```python
from build123d import *

# Parameters (mm, degrees)
BOSS_EXTRUDE1_DEPTH = 40
SKETCH2_R           = 7.5
BOSS_EXTRUDE2_DEPTH = 5
FILLET1_R           = 10


with BuildPart() as part:
    # Sketch1 → Boss-Extrude1 (new, symmetric)
    with BuildSketch(Plane.XY):
        with BuildLine():
            Line((-42.261826174, 90.630778704), (0, 0))
            Line((0, 0), (57.1, 0))
            Line((57.1, 0), (78.545069205, 10))
            Line((78.545069205, 10), (70.06731645, 28.180599453))
            ThreePointArc((70.06731645, 28.180599453), (58.907926391, 38.47561206), (43.733601964, 37.96654498))
            Line((43.733601964, 37.96654498), (15.92675652, 25))
            Line((15.92675652, 25), (-11.151766263, 83.070079506))
            ThreePointArc((-11.151766263, 83.070079506), (-22.437519138, 93.411566687), (-37.730287239, 92.743870012))
            Line((-37.730287239, 92.743870012), (-42.261826174, 90.630778704))
        make_face()
    extrude(amount=BOSS_EXTRUDE1_DEPTH, both=True)

    # Sketch2 → Boss-Extrude2 (add, symmetric)
    with BuildSketch(Plane.XZ):
        with Locations(Location((30, 0, 0), (0, 0, 90))):
            Circle(SKETCH2_R)
    extrude(amount=BOSS_EXTRUDE2_DEPTH, both=True)

    # Fillet1
    # the kernel refuses this fillet: 10 mm, written as the material it takes off along each edge
    with BuildSketch(Plane(origin=(43.733601964, 37.96654498, -40), x_dir=(0.42261826174070133, -0.9063077870366492, 0), z_dir=(-0.9063077870366492, -0.4226182617407013, 0))) as fillet1_piece_1:
        with BuildLine():
            CenterArc((FILLET1_R, FILLET1_R), FILLET1_R, 180, 90)
            Line((0, FILLET1_R), (0, 0))
            Line((0, 0), (FILLET1_R, 0))
        make_face()
    extrude(amount=30.681459259, mode=Mode.SUBTRACT)
    with BuildSketch(Plane(origin=(51.94116071, 19.728234218, -40), x_dir=(0.9063077870366498, 0.42261826174069983, 0), z_dir=(0.42261826174069983, -0.9063077870366498, 0))) as fillet1_piece_2:
        with BuildLine():
            CenterArc((20 - FILLET1_R, FILLET1_R), FILLET1_R, 270, 90)
            Line((20, FILLET1_R), (20, 0))
            Line((20, 0), (20 - FILLET1_R, 0))
        make_face()
    revolve(axis=Axis((51.94116071, 19.728234218, -40), (0, 0, 1)), revolution_arc=89.228578439, mode=Mode.SUBTRACT)
    with BuildSketch(Plane(origin=(89.110525749, -12.657694676, -40), x_dir=(-0.90630778703665, -0.4226182617406995, 0), z_dir=(-0.42261826174069944, 0.9063077870366499, 0))) as fillet1_piece_3:
        with BuildLine():
            CenterArc((FILLET1_R, FILLET1_R), FILLET1_R, 180, 90)
            Line((0, FILLET1_R), (0, 0))
            Line((0, 0), (FILLET1_R, 0))
        make_face()
    extrude(amount=45.06007199, mode=Mode.SUBTRACT)
    with BuildSketch(Plane(origin=(-37.730287239, 92.743870012, -40), x_dir=(0.4226182617406985, -0.9063077870366504, 0), z_dir=(-0.9063077870366504, -0.42261826174069855, 0))) as fillet1_piece_4:
        with BuildLine():
            CenterArc((FILLET1_R, FILLET1_R), FILLET1_R, 180, 90)
            Line((0, FILLET1_R), (0, 0))
            Line((0, 0), (FILLET1_R, 0))
        make_face()
    extrude(amount=30, mode=Mode.SUBTRACT)
    with BuildSketch(Plane(origin=(89.110525749, -12.657694676, 40), x_dir=(-0.90630778703665, -0.4226182617406995, 0), z_dir=(-0.42261826174069944, 0.9063077870366499, 0))) as fillet1_piece_5:
        with BuildLine():
            CenterArc((FILLET1_R, -FILLET1_R), FILLET1_R, 90, 90)
            Line((0, -FILLET1_R), (0, 0))
            Line((0, 0), (FILLET1_R, 0))
        make_face()
    extrude(amount=45.06007199, mode=Mode.SUBTRACT)
    with BuildSketch(Plane(origin=(51.94116071, 19.728234218, 40), x_dir=(0.9063077870366498, 0.42261826174069983, 0), z_dir=(0.42261826174069983, -0.9063077870366498, 0))) as fillet1_piece_6:
        with BuildLine():
            CenterArc((20 - FILLET1_R, -FILLET1_R), FILLET1_R, 0, 90)
            Line((20, -FILLET1_R), (20, 0))
            Line((20, 0), (20 - FILLET1_R, 0))
        make_face()
    revolve(axis=Axis((51.94116071, 19.728234218, 40), (0, 0, 1)), revolution_arc=89.228578439, mode=Mode.SUBTRACT)
    with BuildSketch(Plane(origin=(43.733601964, 37.96654498, 40), x_dir=(0.42261826174070133, -0.9063077870366492, 0), z_dir=(-0.9063077870366492, -0.4226182617407013, 0))) as fillet1_piece_7:
        with BuildLine():
            CenterArc((FILLET1_R, -FILLET1_R), FILLET1_R, 90, 90)
            Line((0, -FILLET1_R), (0, 0))
            Line((0, 0), (FILLET1_R, 0))
        make_face()
    extrude(amount=30.681459259, mode=Mode.SUBTRACT)
    with BuildSketch(Plane(origin=(15.92675652, 25, 40), x_dir=(-0.9063077870366495, -0.42261826174070066, 0), z_dir=(-0.42261826174070066, 0.9063077870366494, 0))) as fillet1_piece_8:
        with BuildLine():
            CenterArc((FILLET1_R, -FILLET1_R), FILLET1_R, 90, 90)
            Line((0, -FILLET1_R), (0, 0))
            Line((0, 0), (FILLET1_R, 0))
        make_face()
    extrude(amount=64.07324348, mode=Mode.SUBTRACT)
    with BuildSketch(Plane(origin=(-29.277922004, 74.617714272, 40), x_dir=(0.9063077870366488, 0.4226182617407019, 0), z_dir=(0.4226182617407019, -0.9063077870366488, 0))) as fillet1_piece_9:
        with BuildLine():
            CenterArc((20 - FILLET1_R, -FILLET1_R), FILLET1_R, 0, 90)
            Line((20, -FILLET1_R), (20, 0))
            Line((20, 0), (20 - FILLET1_R, 0))
        make_face()
    revolve(axis=Axis((-29.277922004, 74.617714272, 40), (0, 0, 1)), revolution_arc=90, mode=Mode.SUBTRACT)
    with BuildSketch(Plane(origin=(-37.730287239, 92.743870012, 40), x_dir=(0.4226182617406985, -0.9063077870366504, 0), z_dir=(-0.9063077870366504, -0.42261826174069855, 0))) as fillet1_piece_10:
        with BuildLine():
            CenterArc((FILLET1_R, -FILLET1_R), FILLET1_R, 90, 90)
            Line((0, -FILLET1_R), (0, 0))
            Line((0, 0), (FILLET1_R, 0))
        make_face()
    extrude(amount=30, mode=Mode.SUBTRACT)
    with BuildSketch(Plane(origin=(-29.277922004, 74.617714272, -40), x_dir=(0.9063077870366488, 0.4226182617407019, 0), z_dir=(0.4226182617407019, -0.9063077870366488, 0))) as fillet1_piece_11:
        with BuildLine():
            CenterArc((20 - FILLET1_R, FILLET1_R), FILLET1_R, 270, 90)
            Line((20, FILLET1_R), (20, 0))
            Line((20, 0), (20 - FILLET1_R, 0))
        make_face()
    revolve(axis=Axis((-29.277922004, 74.617714272, -40), (0, 0, 1)), revolution_arc=90, mode=Mode.SUBTRACT)
    with BuildSketch(Plane(origin=(15.92675652, 25, -40), x_dir=(-0.9063077870366495, -0.42261826174070066, 0), z_dir=(-0.42261826174070066, 0.9063077870366494, 0))) as fillet1_piece_12:
        with BuildLine():
            CenterArc((FILLET1_R, FILLET1_R), FILLET1_R, 180, 90)
            Line((0, FILLET1_R), (0, 0))
            Line((0, 0), (FILLET1_R, 0))
        make_face()
    extrude(amount=64.07324348, mode=Mode.SUBTRACT)
    with BuildSketch(Plane(origin=(43.733601964, 37.96654498, -40), x_dir=(0.42261826174070133, -0.9063077870366492, 0), z_dir=(-0.9063077870366492, -0.4226182617407013, 0))) as fillet1_piece_13a_section:
        with BuildLine():
            CenterArc((FILLET1_R, FILLET1_R), FILLET1_R, 180, 90)
            Line((0, FILLET1_R), (0, 0))
            Line((0, 0), (FILLET1_R, 0))
        make_face()
    fillet1_piece_13a = extrude(amount=55.681459259, mode=Mode.PRIVATE)
    fillet1_piece_13a = split(fillet1_piece_13a, bisect_by=Plane(origin=(16.883543617, 22.94816345, -37.736048857), z_dir=(-0.9063077870366494, -0.42261826174070066, 0)), keep=Keep.TOP, mode=Mode.PRIVATE)
    with BuildSketch(Plane(origin=(26.492213064, 2.342305324, -40), x_dir=(-0.9063077870366495, -0.42261826174070066, 0), z_dir=(-0.42261826174070066, 0.9063077870366494, 0))) as fillet1_piece_13b_section:
        with BuildLine():
            CenterArc((FILLET1_R, FILLET1_R), FILLET1_R, 180, 90)
            Line((0, FILLET1_R), (0, 0))
            Line((0, 0), (FILLET1_R, 0))
        make_face()
    fillet1_piece_13b = extrude(amount=89.07324348, mode=Mode.PRIVATE)
    fillet1_piece_13b = split(fillet1_piece_13b, bisect_by=Plane(origin=(13.87491997, 24.043212903, -37.736048857), z_dir=(0.4226182617407013, -0.9063077870366492, 0)), keep=Keep.TOP, mode=Mode.PRIVATE)
    fillet1_piece_13 = fillet1_piece_13a & fillet1_piece_13b
    add(fillet1_piece_13, mode=Mode.SUBTRACT)
    with BuildSketch(Plane(origin=(43.733601964, 37.96654498, 40), x_dir=(0.42261826174070133, -0.9063077870366492, 0), z_dir=(-0.9063077870366492, -0.4226182617407013, 0))) as fillet1_piece_14a_section:
        with BuildLine():
            CenterArc((FILLET1_R, -FILLET1_R), FILLET1_R, 90, 90)
            Line((0, -FILLET1_R), (0, 0))
            Line((0, 0), (FILLET1_R, 0))
        make_face()
    fillet1_piece_14a = extrude(amount=55.681459259, mode=Mode.PRIVATE)
    fillet1_piece_14a = split(fillet1_piece_14a, bisect_by=Plane(origin=(16.883543617, 22.94816345, 37.736048857), z_dir=(-0.9063077870366494, -0.42261826174070066, 0)), keep=Keep.TOP, mode=Mode.PRIVATE)
    with BuildSketch(Plane(origin=(26.492213064, 2.342305324, 40), x_dir=(-0.9063077870366495, -0.42261826174070066, 0), z_dir=(-0.42261826174070066, 0.9063077870366494, 0))) as fillet1_piece_14b_section:
        with BuildLine():
            CenterArc((FILLET1_R, -FILLET1_R), FILLET1_R, 90, 90)
            Line((0, -FILLET1_R), (0, 0))
            Line((0, 0), (FILLET1_R, 0))
        make_face()
    fillet1_piece_14b = extrude(amount=89.07324348, mode=Mode.PRIVATE)
    fillet1_piece_14b = split(fillet1_piece_14b, bisect_by=Plane(origin=(13.87491997, 24.043212903, 37.736048857), z_dir=(0.4226182617407013, -0.9063077870366492, 0)), keep=Keep.TOP, mode=Mode.PRIVATE)
    fillet1_piece_14 = fillet1_piece_14a & fillet1_piece_14b
    add(fillet1_piece_14, mode=Mode.SUBTRACT)


solid = part.part
```
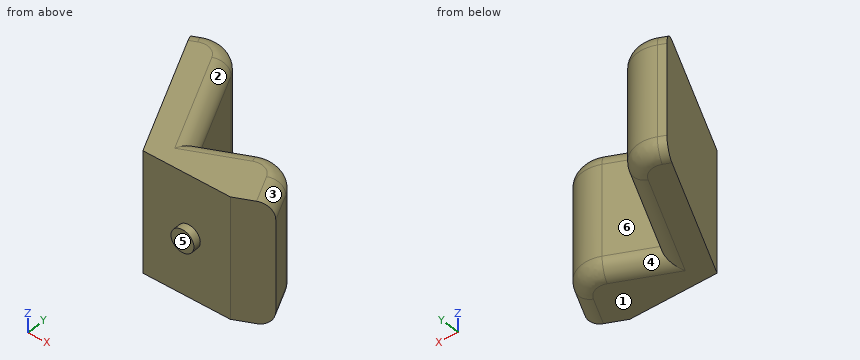
CAD build for the part. Positions are in the model's coordinates, mm. Face numbers are marked on the shaded views. A direction names the side the tool comes from. Give positions to 0.01 mm unless a question says otherwise; leave off trailing zeros. Order: outer loops, then holes, each group sorted by start corner. A loop starts at its lowest first (then second) coordinate and runs counter-clockwise, first axis right, second up. Notation, with made-up numbers: M 69,21 L 83,21 A23 cw 83,44 Z; hole C 19,55.25 d11. An arc over 180 degrees is marked long. Put each result on its own line as item: value. Start each with the question number.
(1) Saw through at A-A, the plane z = 0. Write the cut outline in (x, y).
(2) Drill centre lines: line 1 along X through (y, z) = (34.5, 36); line 2 along Y through (x, z) = (52, 21.5); line 3 along X through (y, z) = (12, 7.5). Where is each one in solid material? Low to high.
(3) Mould opens along X. For the marked faces 1, 2 and 3 say: +X half, -X half, draft (parallel to the pull), parting line (faces both ways), or undercut.
(4) Saw through at B-B, the plane z = 9. Write the cut outline in (x, y), then the cut area to 3 significant figures.
(5) Flat gauge pins, fed straight in: pin 1 Ø8 at (y, z) = (66, 12) entering from -X; pin 2 Ø6 at (x, y) = (-11.5, 13) entering from +Z; pin 3 Ø8 at (x, z) = (-14, -30) entering from -Y; pin 4 Ø4 at (x, z) = (55, -15) entering from +Y. Where does each tip first touch, or does it go through?
(6) Which spindle directions (+Z, -Z, +X, -X, +Y, -Y) get a long thin tool onto all of the face, cutting with end or side? Do the marked faces 4, 5 and 6. Say none if no direction does.
Check result:
1. outline: M -42.26,90.63 L 0,0 L 22.5,0 L 22.5,-5 L 37.5,-5 L 37.5,0 L 57.1,0 L 78.55,10 L 70.07,28.18 A20 ccw 43.73,37.97 L 15.93,25 L -11.15,83.07 A20 ccw -37.73,92.74 Z
2. line 1: x = -16.09 to 9.29, 41.03 to 62.23
2. line 2: y = 0 to 39.73
2. line 3: x = -5.6 to 77.61
3. face 1: draft
3. face 2: undercut
3. face 3: +X half
4. outline: M -42.26,90.63 L 0,0 L 57.1,0 L 78.55,10 L 70.07,28.18 A20 ccw 43.73,37.97 L 15.93,25 L -11.15,83.07 A20 ccw -37.73,92.74 Z
4. area: 4,330 mm2
5. pin 1: stops at x = -32.64
5. pin 2: passes through
5. pin 3: stops at y = 21.45
5. pin 4: stops at y = 39.7
6. face 4: -Z, +Y
6. face 5: +Z, -Z, +X, -X, -Y
6. face 6: +Z, -Z, +Y
